The listing builds one solid part. Answer for the finished solid, in the listing's coordinates (mm). A direction names the side the tool comes from. Coordinates: 2 decimals unless noted, no trailing zeros. Write each loop counter-clockwise with the first axis right and the second up, starting at its lowest first coordinate (ties: lowest second). Pieces come first, ordered by that corner, then holes.
Autodesk Inventor part; units mm, degrees
ref_plane "Work Plane1" through (29, 0, 0) normal (0, -1, 0) x (1, 0, 0)
ref_plane "YZ Plane" through (0, 0, 0) normal (1, 0, 0) x (0, 1, 0)
ref_plane "XZ Plane" through (0, 0, 0) normal (0, 1, 0) x (-1, 0, 0)
sketch "Sketch1" plane through (0, 0, 0) normal (0, 0, 1) x (1, 0, 0)
  line L0 (0.3333, 0) -> (20, 0)
  line L1 (20, 0) -> (20, 2)
  line L2 (20, 2) -> (2.1, 2)
  line L3 (2.1, 2) -> (1.6705, 2)
  line L4 (1.6705, 2) -> (0, 2)
  line L5 (0, 2) -> (0, 3.5)
  line L6 (0, 3.5) -> (-2.8, 3.5)
  line L7 (-2.8, 3.5) -> (-2.8, 1.4434)
  line L8 (-2.8, 1.4434) -> (-0.5, 1.4434)
  line L9 (-0.5, 1.4434) -> (0.3333, 0)
  line L10 (-7.36, 0) -> (24.56, 0)
  line L11 (0, -0.7) -> (0, 4.2)
  line L12 (2.1, 2) -> (0, 2) construction
  dimension "d1" = 17.9
  dimension "d2" = 0.4295
  dimension "d3" = 2.8
  dimension "d4" = 2.3
  dimension "d5" = 60
  dimension "d6" = 4
  dimension "d7" = 4
  dimension "d8" = 2.8868
  dimension "d9" = 7
  dimension "d26" = 20
revolve "Body" add sketch "Sketch1" angle 360 about axis through (0.3333, 0, 0) along (1, 0, 0) contours L9 L11 L4 L3 L2 L1 L0 | L9 L8 L7 L6 L5 L11
sketch "Sketch2" plane through (-2.8, 0, 0) normal (-1, 0, 0) x (0, 0, 1)
  circle A0 centre (0, 0) radius 1.4434
  line L0 (0, -4.9) -> (0, 4.9)
  line L1 (-4.9, 0) -> (4.9, 0)
  line L2 (1.4434, 0) -> (0.7217, -1.25)
  line L3 (0.7217, -1.25) -> (-0.7217, -1.25)
  line L4 (-0.7217, -1.25) -> (-1.4434, 0)
  line L5 (-1.4434, 0) -> (-0.7217, 1.25)
  line L6 (-0.7217, 1.25) -> (0.7217, 1.25)
  line L7 (0.7217, 1.25) -> (1.4434, 0)
  point P0 (0, 0)
extrude "Slot" add sketch "Sketch2" against normal up to next contours L7 A0 | A0 L2 | L6 L0 A0 | A0 L0 L3 | L0 L6 A0 | A0 L3 L0 | L4 A0 | A0 L5
fillet "Fillet1" radius 0.4 1 edges at (-2.8, -3.5, 0)
thread "Thread"
chamfer "Chamfer1" distance 0.4294 distance2 0.4294 1 edges at (20, -2, 0) measured on face at (20, 0.527, -0.2661)
ref_plane "Work Plane1" through (29, 0, 0) normal (0, -1, 0) x (1, 0, 0)
fillet "Fillet2" radius 0.1 1 edges at (0, -2, 0)
equation "\"d1\" = GEL"
equation "\"d3\" = KOH"
equation "\"d4\" = INTI"
equation "\"d6\" = GD"
equation "\"d7\" = BDM"
equation "\"d8\" = 1.1547 * SW"
equation "\"d9\" = KOD"
equation "\"d26\" = NLG"
equation "\"d30\" = R"
equation "\"d17\" = RR"
equation "\"d13\" = GEL"
equation "\"d15\" = -0.5 * SPD + 0.5 * GD"
equation "\"d16\" = GUL"
equation "\"GD\" = NND"
equation "\"NLG\" = 20"
equation "\"GEL\" = 17.9"
equation "\"KOD\" = 7"
equation "\"KOH\" = 2.8"
equation "\"INTI\" = 2.3"
equation "\"GAL\" = 0.61345 * PTC"
equation "\"GUL\" = 0.61345 * PTC"
equation "\"BDM\" = NND"
equation "\"SW\" = 2.5"
equation "\"RR\" = 0.4"
equation "\"SPD\" = NND - 1.2269 * PTC"
equation "\"R\" = 0.1"
equation "\"TOA\" = 30deg"
equation "\"GD1\" = THREADDIA - 1.2269 * PTC"
equation "\"THREADDIA\" = 4"
equation "\"FAWI\" = 45deg"
equation "\"ANG\" = 120deg"
equation "\"PTC\" = 0.7"
equation "\"NND\" = 4"
equation "\"E0\" = 1.155 * SW"
properties part number "DIN 7984 - M4 x 20" material "Steel, Mild"
Q1. Determine the mould class of faces 4 (the face through (10, 0, 2)), 5 (the face through (-2.8, -0.6, 1.3)), 6 (the face through (-2, -1.25, 0)) for opening direction Y: released by +Y, released by -Y, zero draft, split by the parting line, or undercut.
Answers below:
face 4: split by the parting line
face 5: zero draft
face 6: undercut
Q2. Given pin 1 (4 mm diameter, centred on x = 1.5, z = 3, fed in from +Y); pin 2 (1.5 mm diameter, centred on x = 6.5, z = 1.5, fed in from +Y); pin 3 (2 mm diameter, centred on x = 5.5, y = 1.5, fed in from +Z), each flat-ended and moving along its own axis, determine where each tip first touches the part or whether it passes through.
Answers below:
pin 1: stops at y = 3.07
pin 2: stops at y = 1.85
pin 3: stops at z = 1.94
Q3. Find the intervals of material crossed by probe 1 along X at (y, z) = (0.75, -2); probe 2 along Y at (x, z) = (16.25, 0.75); probe 3 along X at (y, z) = (-1.5, -0.5), in increasing order.
Answers below:
probe 1: x = -2.8 to 0
probe 2: y = -1.85 to 1.85
probe 3: x = -2.8 to 19.99
Q4. Which of the six approach directions +Z, -Z, +X, -X, +Y, -Y give full straight-line access (tool end or side, diameter ignored) to faces 1 (the face through (-1.611, -0.616, 1.088)), 2 (the face through (0, 2, -2)), 3 (the face through (-1.217, 3.233, 1.341))?
Answers below:
face 1: -X
face 2: +X
face 3: +X, -X
Q5. The part is cut by section A-A, the plane x = 5.75. Write down the section's boundary in (y, z).
Answers below:
outline: circle Ø4 at (0, 0)
